Check sheet for the modelled part. Datum: model origin and axes. Units: mm. A direction names the side the tool comes from. Coordinates: 2 decimals unless noted, no trailing zeros. Order: outer loops, then holes, each group sorted by start corner. A loop starts at its lowest first (then second) coordinate and runs counter-clockwise, first axis right, second up.
1. Cross-section at D-D (z = 14.5). Enter the section's corners in (x, y), then the cut area to 3 significant figures.
2. Cross-section at C-C (y = 76.5). Count the separate pieces of the cut face and the enclosed holes in it, then the cut area to 3 significant figures.
3. Cross-section at B-B (z = -22). Enter the section's corners in (x, y).
4. Set-up check for faces 4 (the flat face through (-25, 83, 3)), 5 (the cylindrical face through (10.72, 60.51, -9.45)), 6 (the cylindrical face through (-5.46, 74.45, 0.34)): record each of +Z, -Z, +X, -X, +Y, -Y from which the full face is reachable in a straight line by a thin tool's end or side.
5. Draft check along Z on faces 1 (the cylindrical face through (1.32, 53.46, 29.97)), 2 (the cylindrical face through (9.77, 55.01, -19.09)), 3 (the flat face through (0, 56, -15)). Enter one of: released by +Z, released by -Z, zero draft, split by the parting line, or undercut.
6. Gauge pin test, flat ends, axial feed: pin 1 Ø1.9 at (x, y) = (-5.5, 126.5) entering from +Z; pin 2 Ø2 at (y, z) = (90, -8.5) entering from +X; pin 3 Ø2.5 at (x, y) = (5, 76.5) entering from -Z; pin 4 Ø3 at (x, z) = (-17.5, -23) entering from +Y. Record the tip position at first contact, or that the pin passes through.
7. Cross-section at A-A (y = 99). Enter the section's corners in (x, z), then the cut area to 3 significant figures.
8. Thickness scan on line 1 (X direction, y = 85, z = 11.5); line 2 (X direction, y = 53.35, z = -23); line 3 (X direction, y = 55, z = -23). Record the ranges inside material, lowest first.
```python
from build123d import *

# Parameters (mm, degrees)
BOSS_EXTRUDE1_DEPTH = 16
CHAMFER1_SIZE       = 5
CUT_EXTRUDE1_DEPTH  = 10.25
SKETCH5_W           = 6.4
SKETCH5_H           = 6.71
CUT_EXTRUDE2_DEPTH  = 24
CUT_EXTRUDE3_DEPTH  = 10
FILLET1_R           = 15
CHAMFER2_SIZE       = 3
SKETCH7_R           = 30
SKETCH7_R_2         = 2
BOSS_EXTRUDE2_DEPTH = 5
SKETCH8_R           = 4.5
CUT_EXTRUDE4_DEPTH  = 2


# Some blends are built 0.0001 mm under size
with BuildPart() as part:
    # Sketch1 → Boss-Extrude1 (new, symmetric)
    with BuildSketch(Plane.XY):
        with BuildLine():
            Line((25, 51), (-25, 51))
            Line((-25, 51), (-25, 111))
            ThreePointArc((-25, 111), (0, 136), (25, 111))
            Line((25, 111), (25, 51))
        make_face()
    extrude(amount=BOSS_EXTRUDE1_DEPTH, both=True)

    # Chamfer1
    chamfer1_edges = [part.edges().sort_by_distance(p)[0] for p in [
        (25, 81, -16),
        (-25, 81, -16),
        (0, 136, -16),
    ]]
    chamfer(chamfer1_edges, length=CHAMFER1_SIZE)

    # Sketch3 → Cut-Extrude1 (cut, symmetric)
    with BuildSketch(Plane(origin=(0, 0, 0), x_dir=(0, 0, -1), z_dir=(1, 0, 0))):
        Polygon((-3.3, 121.79), (-3.3, 131.5), (-16, 131.5), (-16, 101.5), (16, 101.5), (16, 121.79), align=None)
    cut_extrude1 = extrude(amount=CUT_EXTRUDE1_DEPTH, both=True, mode=Mode.SUBTRACT)

    # Sketch4 → Cut-Revolve1 (revolve, cut)
    with BuildSketch(Plane(origin=(-5, 0, 0), x_dir=(0, 0, -1), z_dir=(1, 0, 0)), mode=Mode.PRIVATE) as cut_revolve1_sk:
        Polygon((-3.3, 126.5), (6.7, 126.5), (6.7, 127.85), (2.7, 127.85), (2.7, 128.6), (-3.3, 128.6), align=None)
    cut_revolve1 = revolve(cut_revolve1_sk.sketch.rotate(Axis((-5, 126.5, 3.3), (0, 0, -1)), 90), axis=Axis((-5, 126.5, 3.3), (0, 0, -1)), mode=Mode.SUBTRACT)

    # Mirror1: Cut-Revolve1 across plane
    add(cut_revolve1.mirror(Plane(origin=(0, 0, 0), x_dir=(0, 0, 1), z_dir=(1, 0, 0))), mode=Mode.SUBTRACT)

    # Mirror2: Cut-Extrude1, Cut-Revolve1 across plane
    add(cut_extrude1.mirror(Plane(origin=(-10.25, 101.5, -16), x_dir=(0, 0, 1), z_dir=(0, -1, 0))), mode=Mode.SUBTRACT)
    add(cut_revolve1.mirror(Plane(origin=(-10.25, 101.5, -16), x_dir=(0, 0, 1), z_dir=(0, -1, 0))), mode=Mode.SUBTRACT)

    # Mirror2 copy 1 sketch → Mirror2 copy 1 (revolve, cut)
    with BuildSketch(Plane(origin=(5, 203, 0), x_dir=(0, 0, -1), z_dir=(-1, 0, 0))):
        Polygon((-3.3, 126.5), (6.7, 126.5), (6.7, 127.85), (2.7, 127.85), (2.7, 128.6), (-3.3, 128.6), align=None)
    revolve(axis=Axis((5, 76.5, 3.3), (0, 0, -1)), mode=Mode.SUBTRACT)

    # Sketch5 → Cut-Extrude2 (cut)
    with BuildSketch(Plane.XY.offset(3.3)):
        with Locations((0, 125.145)):
            Rectangle(SKETCH5_W, SKETCH5_H)
    extrude(amount=-CUT_EXTRUDE2_DEPTH, mode=Mode.SUBTRACT)

    # Sketch6 → Cut-Extrude3 (cut)
    with BuildSketch(Plane(origin=(0, 0, -16), x_dir=(-1, 0, 0), z_dir=(0, 0, -1))):
        with BuildLine():
            Line((-15, 111), (-15, 56))
            Line((-15, 56), (15, 56))
            Line((15, 56), (15, 111))
            ThreePointArc((15, 111), (0, 126), (-15, 111))
        make_face()
    extrude(amount=-CUT_EXTRUDE3_DEPTH, mode=Mode.SUBTRACT)

    # Fillet1
    fillet1_edges = [part.edges().sort_by_distance(p)[0] for p in [
        (-15, 56, -11),
        (15, 56, -11),
    ]]
    fillet(fillet1_edges, radius=FILLET1_R - 0.0001)  # a hair under: the kernel refuses the full size

    # Chamfer2
    # the kernel refuses this chamfer: 3 mm, written as the material it takes off along each edge
    with BuildSketch(Plane(origin=(-15, 70.9999, -16), x_dir=(-0.9996219169112965, 0, -0.02749587661058676), z_dir=(0, 1, 0)), Plane(origin=(15, 111, -16), x_dir=(0.9996219169112965, 0, -0.02749587661058676), z_dir=(0, -1, 0))) as chamfer2_piece_1:
        Polygon((CHAMFER2_SIZE * 0.999621916911, CHAMFER2_SIZE * 0.0274958766106), (-CHAMFER2_SIZE * 0.0274958766106, CHAMFER2_SIZE * 0.999621916911), (0, 0), align=None)
    extrude(amount=40.0001, mode=Mode.SUBTRACT)
    with BuildSketch(Plane(origin=(-0.0001, 70.9999, -16), x_dir=(0, -1, 0), z_dir=(1, 0, 0))) as chamfer2_piece_2:
        Polygon((14.9999 + CHAMFER2_SIZE, 0), (14.9999, -CHAMFER2_SIZE), (14.9999, 0), align=None)
    revolve(axis=Axis((-0.0001, 70.9999, -16), (0, 0, -1)), revolution_arc=90, mode=Mode.SUBTRACT)
    with BuildSketch(Plane(origin=(0, 111, -16), x_dir=(-0.29504722278554535, 0.955482671913278, 0), z_dir=(-0.955482671913278, -0.29504722278554535, 0))) as chamfer2_piece_3:
        Polygon((15 + CHAMFER2_SIZE, 0), (15, -CHAMFER2_SIZE), (15, 0), align=None)
    revolve(axis=Axis((0, 111, -16), (0, 0, -1)), revolution_arc=107.160369077, mode=Mode.SUBTRACT)
    with BuildSketch(Plane(origin=(0.0001, 70.9999, -16), x_dir=(1, 0, 0), z_dir=(0, 1, 0))) as chamfer2_piece_4:
        Polygon((14.9999 + CHAMFER2_SIZE, 0), (14.9999, -CHAMFER2_SIZE), (14.9999, 0), align=None)
    revolve(axis=Axis((0.0001, 70.9999, -16), (0, 0, -1)), revolution_arc=90, mode=Mode.SUBTRACT)
    with BuildSketch(Plane(origin=(0.0001, 56, -16), x_dir=(0, -0.9996219169112965, -0.02749587661058676), z_dir=(-1, 0, 0))) as chamfer2_piece_5:
        Polygon((CHAMFER2_SIZE * 0.999621916911, CHAMFER2_SIZE * 0.0274958766106), (-CHAMFER2_SIZE * 0.0274958766106, CHAMFER2_SIZE * 0.999621916911), (0, 0), align=None)
    extrude(amount=0.0002, mode=Mode.SUBTRACT)
    with BuildSketch(Plane(origin=(0, 111, -16), x_dir=(-1, 0, 0), z_dir=(0, -1, 0))) as chamfer2_piece_6:
        Polygon((15 + CHAMFER2_SIZE, 0), (15, -CHAMFER2_SIZE), (15, 0), align=None)
    revolve(axis=Axis((0, 111, -16), (0, 0, -1)), revolution_arc=107.160369077, mode=Mode.SUBTRACT)

    # Sketch7 → Boss-Extrude2 (add)
    with BuildSketch(Plane.XZ.offset(-51)):
        with Locations(Location((0, 0, 0), (0, 0, 270))):
            Circle(SKETCH7_R)
        with Locations(Location((-12, -23, 0), (0, 0, 270))):
            Circle(SKETCH7_R_2, mode=Mode.SUBTRACT)
        with Locations(Location((12, -23, 0), (0, 0, 270))):
            Circle(SKETCH7_R_2, mode=Mode.SUBTRACT)
        with Locations(Location((-12, 23, 0), (0, 0, 270))):
            Circle(SKETCH7_R_2, mode=Mode.SUBTRACT)
        with Locations(Location((12, 23, 0), (0, 0, 270))):
            Circle(SKETCH7_R_2, mode=Mode.SUBTRACT)
    extrude(amount=-BOSS_EXTRUDE2_DEPTH)

    # Sketch8 → Cut-Extrude4 (cut)
    with BuildSketch(Plane(origin=(0, 56, 0), x_dir=(1, 0, 0), z_dir=(0, 1, 0))):
        with Locations((12, 23)):
            Circle(SKETCH8_R)
        with Locations((-12, 23)):
            Circle(SKETCH8_R)
        with Locations((-12, -23)):
            Circle(SKETCH8_R)
        with Locations((12, -23)):
            Circle(SKETCH8_R)
    extrude(amount=-CUT_EXTRUDE4_DEPTH, mode=Mode.SUBTRACT)


solid = part.part
```
Data:
1. outline: (-26.26, 51) - (26.26, 51) - (26.26, 56) - (25, 56) - (25, 111) arc R25 ccw to (-25, 111) - (-25, 56) - (-26.26, 56) - close; hole (-10.25, 71.5) - (10.25, 71.5) - (10.25, 131.5) - (-10.25, 131.5) - close
1. area: 2,760 mm2
2. separate pieces: 3
2. enclosed holes: 0
2. area: 937 mm2
3. outline: (-20.4, 51) - (-13.73, 51) - (-13.73, 54) - (-16.39, 54) - (-16.39, 56) - (-20.4, 56) - close; (-10.27, 51) - (10.27, 51) - (10.27, 54) - (7.61, 54) - (7.61, 56) - (-7.61, 56) - (-7.61, 54) - (-10.27, 54) - close; (13.73, 51) - (20.4, 51) - (20.4, 56) - (16.39, 56) - (16.39, 54) - (13.73, 54) - close
4. face 4: +Z, -Z, -X, +Y
4. face 5: -Z
4. face 6: +Z
5. face 1: split by the parting line
5. face 2: undercut
5. face 3: zero draft
6. pin 1: stops at z = -2.7
6. pin 2: stops at x = 25
6. pin 3: passes through
6. pin 4: stops at y = 56
7. outline: (-25, -11) - (-20, -16) - (-18, -16) - (-15, -13) - (-15, -6) - (-10.25, -6) - (-10.25, 16) - (-25, 16) - close; (10.25, -6) - (15, -6) - (15, -13) - (18, -16) - (20, -16) - (25, -11) - (25, 16) - (10.25, 16) - close
7. area: 815 mm2
8. line 1: x = -25 to -10.25, 10.25 to 25
8. line 2: x = -19.26 to -14, -10 to 10, 14 to 19.26
8. line 3: x = -19.26 to -16.5, -7.5 to 7.5, 16.5 to 19.26
